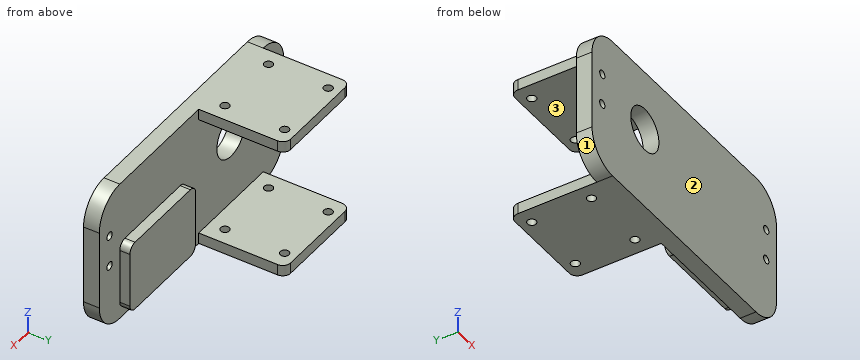
```python
from build123d import *

# Parameters (mm, degrees)
SKETCH1_W           = 228.6
SKETCH1_H           = 114.78
BOSS_EXTRUDE1_DEPTH = 12.7
SKETCH2_W           = 80.01
SKETCH2_H           = 8.89
BOSS_EXTRUDE2_DEPTH = 69.85
SKETCH3_W           = 81.28
SKETCH3_H           = 57
BOSS_EXTRUDE3_DEPTH = 8.159375
SKETCH4_R           = 17.4625
CUT_EXTRUDE1_DEPTH  = 146.729628422
SKETCH5_R           = 3.4925
CUT_EXTRUDE2_DEPTH  = 182.80605298
SKETCH6_R           = 17.4625
SKETCH6_R_2         = 3.25
CUT_EXTRUDE3_DEPTH  = 146.729628422
FILLET1_R           = 25.4
FILLET2_R           = 6.35
FILLET3_R           = 6.35


with BuildPart() as part:
    # Sketch1 → Boss-Extrude1 (new body)
    with BuildSketch(Plane(origin=(0, 0, 0), x_dir=(1, 0, 0), z_dir=(0, 1, 0))):
        Rectangle(SKETCH1_W, SKETCH1_H)
    extrude(amount=BOSS_EXTRUDE1_DEPTH)

    # Sketch2 → Boss-Extrude2 (add)
    with BuildSketch(Plane(origin=(0, 12.7, 0), x_dir=(1, 0, 0), z_dir=(0, 1, 0))):
        with Locations((-48.895, 52.945)):
            Rectangle(SKETCH2_W, SKETCH2_H)
        with Locations((-48.895, -52.945)):
            Rectangle(SKETCH2_W, SKETCH2_H)
    extrude(amount=BOSS_EXTRUDE2_DEPTH)

    # Sketch3 → Boss-Extrude3 (add)
    with BuildSketch(Plane(origin=(0, 12.7, 0), x_dir=(1, 0, 0), z_dir=(0, 1, 0))):
        with Locations((48.26, 21.5)):
            Rectangle(SKETCH3_W, SKETCH3_H)
    extrude(amount=BOSS_EXTRUDE3_DEPTH)

    # Sketch4 → Cut-Extrude1 (cut, through all)
    with BuildSketch(Plane(origin=(0, 12.7, 0), x_dir=(1, 0, 0), z_dir=(0, 1, 0))):
        with Locations(Location((-48.9, -8.5, 0), (0, 0, 270))):
            Circle(SKETCH4_R)
    extrude(amount=-CUT_EXTRUDE1_DEPTH, mode=Mode.SUBTRACT)

    # Sketch5 → Cut-Extrude2 (cut, through all)
    with BuildSketch(Plane.XY.offset(57.39)):
        with Locations((-75.946, 73.359375)):
            Circle(SKETCH5_R)
        with Locations((-21.946, 73.359375)):
            Circle(SKETCH5_R)
        with Locations((-75.946, 25.359375)):
            Circle(SKETCH5_R)
        with Locations((-21.946, 25.359375)):
            Circle(SKETCH5_R)
    extrude(amount=-CUT_EXTRUDE2_DEPTH, mode=Mode.SUBTRACT)

    # Sketch6 → Cut-Extrude3 (cut, through all)
    with BuildSketch(Plane(origin=(0, 12.7, 0), x_dir=(1, 0, 0), z_dir=(0, 1, 0))):
        with Locations(Location((-48.9, -8.5, 0), (0, 0, 270))):
            Circle(SKETCH6_R)
        with Locations(Location((-101.6, -21.2, 0), (0, 0, 270))):
            Circle(SKETCH6_R_2)
        with Locations(Location((-101.6, 4.2, 0), (0, 0, 270))):
            Circle(SKETCH6_R_2)
        with Locations(Location((101.6, -21.2, 0), (0, 0, 270))):
            Circle(SKETCH6_R_2)
        with Locations(Location((101.6, 4.2, 0), (0, 0, 270))):
            Circle(SKETCH6_R_2)
    extrude(amount=-CUT_EXTRUDE3_DEPTH, mode=Mode.SUBTRACT)

    # Fillet1
    fillet1_edges = [part.edges().sort_by_distance(p)[0] for p in [
        (114.3, 6.35, 57.39),
        (-114.3, 6.35, 57.39),
        (-114.3, 6.35, -57.39),
        (114.3, 6.35, -57.39),
    ]]
    fillet(fillet1_edges, radius=FILLET1_R)

    # Fillet2
    fillet2_edges = [part.edges().sort_by_distance(p)[0] for p in [
        (-88.9, 82.55, -52.945),
        (-8.89, 82.55, -52.945),
        (-88.9, 82.55, 52.945),
        (-8.89, 82.55, 52.945),
    ]]
    fillet(fillet2_edges, radius=FILLET2_R)

    # Fillet3
    fillet3_edges = [part.edges().sort_by_distance(p)[0] for p in [
        (88.9, 16.7796875, 7),
        (88.9, 16.7796875, -50),
        (7.62, 16.7796875, -50),
        (7.62, 16.7796875, 7),
    ]]
    fillet(fillet3_edges, radius=FILLET3_R)


solid = part.part
```
The model under review builds one solid part; all positions refer to its coordinate system, in mm. Face numbers are marked on the shaded views. Round coordinates to 2 decimals unless told otherwise and drop trailing zeros. Loops run counter-clockwise (first coordinate to the right, second up) from the corner with the lowest first, then second, coordinate; pieces in that order, holes last. Notation, with made-up numbers: (6.5, 88.5) -> (21.5, 88.5) arc R21 ccw to (21.5, 104.5) -> close; hole circle Ø11 at (47, 67.25). An arc over 180 degrees is marked (long way). Answer as a JSON object with one key per item and string values. Group by question number.
1) We need section C-C on z = 21.5. Write out the cut boundary in (x, y).
2) We need section D-D on z = -14. Write out the cut boundary in (x, y), then the cut area to 3 significant figures.
3) For line 1 (Y direction, x = -78, z = -49); line 2 (Z direction, x = -47, y = 15); line 3 (Y direction, x = -7.5, z = 29), list the stretches that pass through material, from the lowest coordinate up. Write a range as [from, to].
4) For pin 1 Ø7 at (y, z) = (46, -54.5) entering from -X; pin 2 Ø6 at (x, z) = (-101.6, -4.2) entering from +Y; pin 3 Ø3 at (x, z) = (69, 19) entering from +Y; pin 4 Ø4 at (y, z) = (16, -10.5) entering from +X, all flat-tipped, find the tip position at first contact; note any pin that passes through.
5) We need section B-B on x = -48.9. Write out the cut boundary in (y, z).
6) Mouldability with a two-part tool opening along Z and no side actions: class the marked faces 1, 2 and 3 as released by +Z, released by -Z, zero draft, split by the parting line, or undercut.
7) We need section A-A on y = 44. Write out the cut boundary in (x, z), then the cut area to 3 significant figures.
Result set:
{
 "1": {"outline": "(-114.3, 0) -> (-104.84, 0) -> (-104.84, 12.7) -> (-114.3, 12.7) -> close; (-98.36, 0) -> (-60.56, 0) -> (-60.56, 12.7) -> (-98.36, 12.7) -> close; (-37.24, 0) -> (98.36, 0) -> (98.36, 12.7) -> (-37.24, 12.7) -> close; (104.84, 0) -> (114.3, 0) -> (114.3, 12.7) -> (104.84, 12.7) -> close"},
 "2": {"outline": "(-114.3, 0) -> (114.3, 0) -> (114.3, 12.7) -> (88.9, 12.7) -> (88.9, 20.86) -> (7.62, 20.86) -> (7.62, 12.7) -> (-114.3, 12.7) -> close", "area": "3,570 mm²"},
 "3": {"line 1": "[0, 22.53], [28.18, 70.53], [76.18, 82.55]", "line 2": "[-57.39, -48.5], [48.5, 57.39]", "line 3": "[0, 12.7]"},
 "4": {"pin 1": "x = -88.9", "pin 2": "through", "pin 3": "y = 12.7", "pin 4": "x = 88.9"},
 "5": {"outline": "(0, -57.39) -> (82.55, -57.39) -> (82.55, -48.5) -> (12.7, -48.5) -> (12.7, -8.96) -> (0, -8.96) -> close; (0, 25.96) -> (12.7, 25.96) -> (12.7, 48.5) -> (82.55, 48.5) -> (82.55, 57.39) -> (0, 57.39) -> close"},
 "6": {"face 1": "released by -Z", "face 2": "zero draft", "face 3": "undercut"},
 "7": {"outline": "(-88.9, -57.39) -> (-8.89, -57.39) -> (-8.89, -48.5) -> (-88.9, -48.5) -> close; (-88.9, 48.5) -> (-8.89, 48.5) -> (-8.89, 57.39) -> (-88.9, 57.39) -> close", "area": "1,420 mm²"}
}
